Here's how the part is built. I have some questions about the finished solid (model axes, mm). Round coordinates to 2 decimals unless told otherwise and drop trailing zeros. Loops run counter-clockwise (first coordinate to the right, second up) from the corner with the lowest first, then second, coordinate; pieces in that order, holes last. Notation, with made-up numbers: M -28,-8 L 2,-8 A16 cw 2,2 Z; hole C 81,-31 d6. An arc over 180 degrees is marked long. Answer as a JSON object with one key per item and string values.
from build123d import *

# Parameters (mm, degrees)
SKETCH1_R                    = 50
BOSS_EXTRUDE1_DEPTH          = 5
F_25_0_25_DIAMETER_HOLE1_D   = 25
F_10_2_10_2_DIAMETER_HOLE1_D = 10.2
M3_CLEARANCE_HOLE1_D         = 3.4
M3_CLEARANCE_HOLE2_D         = 3.4
SKETCH11_R                   = 1.5
CUT_EXTRUDE1_DEPTH           = 10
SKETCH12_R                   = 4
CUT_EXTRUDE2_DEPTH           = 10


with BuildPart() as part:
    # Sketch1 → Boss-Extrude1 (new body)
    with BuildSketch(Plane.XY):
        Circle(SKETCH1_R)
    extrude(amount=BOSS_EXTRUDE1_DEPTH)

    # Ø25.0 (25) Diameter Hole1 (through all)
    with Locations(Plane(origin=(0, 0, 0), x_dir=(-1, 0, 0), z_dir=(0, 0, -1))):
        with Locations((0, 0)):
            Hole(F_25_0_25_DIAMETER_HOLE1_D / 2)

    # Ø10.2 (10.2) Diameter Hole1 (through all)
    with Locations(Plane(origin=(0, 0, 0), x_dir=(-1, 0, 0), z_dir=(0, 0, -1))):
        with Locations((37, 0), (-37, 0), (0, -40)):
            Hole(F_10_2_10_2_DIAMETER_HOLE1_D / 2)

    # M3 Clearance Hole1 (through all)
    with Locations(Plane.XY.offset(5)):
        with Locations((46, 0), (28, 0), (9, -40), (-9, -40), (-46, 0), (-28, 0)):
            Hole(M3_CLEARANCE_HOLE1_D / 2)

    # M3 Clearance Hole2 (through all)
    with Locations(Plane.XY.offset(5)):
        with Locations((15.5, 15.5), (15.5, -15.5), (-15.5, -15.5), (-15.5, 15.5)):
            Hole(M3_CLEARANCE_HOLE2_D / 2)

    # Sketch11 → Cut-Extrude1 (cut)
    with BuildSketch(Plane.XY.offset(5)):
        with Locations((-10, 27)):
            Circle(SKETCH11_R)
        with Locations((10, 27)):
            Circle(SKETCH11_R)
    extrude(amount=-CUT_EXTRUDE1_DEPTH, mode=Mode.SUBTRACT)

    # Sketch12 → Cut-Extrude2 (cut)
    with BuildSketch(Plane.XY.offset(5)):
        with Locations((28.284271247, 28.284271247)):
            Circle(SKETCH12_R)
    extrude(amount=-CUT_EXTRUDE2_DEPTH, mode=Mode.SUBTRACT)


solid = part.part
Item 1: I want a section at C-C, the plane x = -28. Please give me the cut outline in (y, z), then the cut area to 3 significant figures.
Resolved:
{"outline": "M -41.42,0 L -1.7,0 L -1.7,5 L -41.42,5 Z; M 1.7,0 L 41.42,0 L 41.42,5 L 1.7,5 Z", "area": "397 mm²"}
Item 2: I'm going to push flat-ended pins straight in: pin 1 Ø4.5 at (x, y) = (-15.5, 15.5) entering from -Z; pin 2 Ø1 at (x, z) = (27.5, 3) entering from -Y; pin 3 Ø3 at (y, z) = (20, 2) entering from -X; pin 4 Ø1 at (x, z) = (-15.5, 2.5) entering from +Y. Where does each tip first touch, or does it pass through?
Resolved:
{"pin 1": "z = 0", "pin 2": "y = -42.08", "pin 3": "x = -46.45", "pin 4": "y = 47.7"}
Item 3: I want a section at D-D, the plane y = 10.5. Please give me the cut outline in (x, z), then the cut area to 3 significant figures.
Resolved:
{"outline": "M -48.89,0 L -6.78,0 L -6.78,5 L -48.89,5 Z; M 6.78,0 L 48.89,0 L 48.89,5 L 6.78,5 Z", "area": "421 mm²"}
Item 4: Please list where these lines run through material, in increasing order: probe 1 along Y at (x, z) = (10, 2); probe 2 along Y at (x, z) = (28, 3.95); probe 3 along Y at (x, z) = (27, 3.3). Write a range as from..to.
Resolved:
{"probe 1": "-48.99..-41.37, -38.63..-7.5, 7.5..25.5, 28.5..48.99", "probe 2": "-41.42..-1.7, 1.7..24.29, 32.27..41.42", "probe 3": "-42.08..-1.37, 1.37..24.5, 32.07..42.08"}
Item 5: If we mould it in two halves opening along X, with no side actions, what happens to faces 1 (the face through (47.7, 0.07, 2.47)), 2 (the face through (47.69, 15.02, 2.46)), 3 (the face through (10, -10, 5))? For each: pulls with the +X half, pulls with the -X half, needs draft (parallel to the pull), parting line crosses it, or undercut.
Resolved:
{"face 1": "undercut", "face 2": "parting line crosses it", "face 3": "needs draft"}
Item 6: I want a section at A-A, the plane x = 0. Please give me the cut outline in (y, z), then the cut area to 3 significant figures.
Resolved:
{"outline": "M -50,0 L -45.1,0 L -45.1,5 L -50,5 Z; M -34.9,0 L -12.5,0 L -12.5,5 L -34.9,5 Z; M 12.5,0 L 50,0 L 50,5 L 12.5,5 Z", "area": "324 mm²"}
Item 7: I want a section at B-B, the plane y = 27. Please give me the cut outline in (x, z), then the cut area to 3 significant figures.
Resolved:
{"outline": "M -42.08,0 L -11.5,0 L -11.5,5 L -42.08,5 Z; M -8.5,0 L 8.5,0 L 8.5,5 L -8.5,5 Z; M 11.5,0 L 24.5,0 L 24.5,5 L 11.5,5 Z; M 32.07,0 L 42.08,0 L 42.08,5 L 32.07,5 Z", "area": "353 mm²"}
